Part model, mm, in its own coordinate system. A direction names the side the tool comes from. Round coordinates to 2 decimals unless told otherwise and drop trailing zeros. Write each loop counter-clockwise with the first axis right and the second up, starting at its lowest first coordinate (ties: lowest second). Pieces come first, ordered by that corner, then holes. Notation, with made-up numbers: (-38.5, 87) -> (7.5, 87) arc R9 cw to (7.5, 92) -> close; hole circle Ø7 at (39.25, -15). An arc over 180 degrees is marked (long way). Return JSON: item names as keys, results as strings. Group by question number.
```python
from build123d import *

# Parameters (mm, degrees)
SKETCH3_W           = 83
SKETCH3_H           = 60
BOSS_EXTRUDE1_DEPTH = 3
SKETCH4_R           = 1.5
CUT_EXTRUDE1_DEPTH  = 3
FILLET2_R           = 3
FILLET3_R           = 3
SKETCH8_R           = 2
BOSS_EXTRUDE2_DEPTH = 6
FILLET4_R           = 3
SKETCH9_R           = 0.3
CUT_EXTRUDE2_DEPTH  = 3


with BuildPart() as part:
    # Sketch3 → Boss-Extrude1 (new body)
    with BuildSketch(Plane(origin=(0, 0, 0), x_dir=(1, 0, 0), z_dir=(0, 1, 0))):
        Rectangle(SKETCH3_W, SKETCH3_H)
    extrude(amount=BOSS_EXTRUDE1_DEPTH)

    # Sketch4 → Cut-Extrude1 (cut)
    with BuildSketch(Plane(origin=(0, 3, 0), x_dir=(1, 0, 0), z_dir=(0, 1, 0))):
        with Locations(Location((-36.5, 25, 0), (0, 0, 270))):
            Circle(SKETCH4_R)
        with Locations(Location((36.5, 25, 0), (0, 0, 270))):
            Circle(SKETCH4_R)
        with Locations(Location((36.5, -25, 0), (0, 0, 270))):
            Circle(SKETCH4_R)
        with Locations(Location((-36.5, -25, 0), (0, 0, 270))):
            Circle(SKETCH4_R)
    extrude(amount=-CUT_EXTRUDE1_DEPTH, mode=Mode.SUBTRACT)

    # Fillet2
    fillet2_edges = [part.edges().sort_by_distance(p)[0] for p in [
        (-41.5, 1.5, 30),
    ]]
    fillet(fillet2_edges, radius=FILLET2_R)

    # Fillet3
    fillet3_edges = [part.edges().sort_by_distance(p)[0] for p in [
        (-41.5, 1.5, -30),
        (41.5, 1.5, -30),
        (41.5, 1.5, 30),
    ]]
    fillet(fillet3_edges, radius=FILLET3_R)

    # Sketch8 → Boss-Extrude2 (add)
    with BuildSketch(Plane(origin=(0, 0, 0), x_dir=(-1, 0, 0), z_dir=(0, -1, 0))):
        with Locations(Location((27.892503865, -25.595481363, 0), (0, 0, 90))):
            Circle(SKETCH8_R)
        with Locations(Location((-32.019288728, -24.830385061, 0), (0, 0, 90))):
            Circle(SKETCH8_R)
        with Locations(Location((-32.019288728, 24.653970247, 0), (0, 0, 90))):
            Circle(SKETCH8_R)
        with Locations(Location((27.892503865, 24.404518637, 0), (0, 0, 90))):
            Circle(SKETCH8_R)
    extrude(amount=BOSS_EXTRUDE2_DEPTH)

    # Fillet4
    fillet4_edges = [part.edges().sort_by_distance(p)[0] for p in [
        (-27.892503865, 0, -22.404518637),
    ]]
    fillet(fillet4_edges, radius=FILLET4_R)
    fillet4_2_edges = [part.edges().sort_by_distance(p)[0] for p in [
        (-27.892503865, 0, 27.595481363),
    ]]
    fillet(fillet4_2_edges, radius=FILLET4_R)
    # the kernel refuses this fillet: 3 mm, written as the material it adds along each edge
    with BuildSketch(Plane(origin=(32.019288728, 0, 24.830385061), x_dir=(0, 0, -1), z_dir=(-1, 0, 0))) as fillet4_3_piece_1_section:
        with BuildLine():
            CenterArc((2 + FILLET4_R, FILLET4_R), FILLET4_R, 180, 90)
            Line((2, FILLET4_R), (2 - FILLET4_R * 0.02, FILLET4_R))
            Line((2 - FILLET4_R * 0.02, FILLET4_R), (2 - FILLET4_R * 0.02, -FILLET4_R * 0.02))
            Line((2 - FILLET4_R * 0.02, -FILLET4_R * 0.02), (2 + FILLET4_R, -FILLET4_R * 0.02))
            Line((2 + FILLET4_R, -FILLET4_R * 0.02), (2 + FILLET4_R, 0))
        make_face()
    fillet4_3_piece_1 = revolve(axis=Axis((32.019288728, 0, 24.830385061), (0, -1, 0)), mode=Mode.PRIVATE)
    fillet4_3_piece_1 = fillet4_3_piece_1 - Plane(origin=(36.5, -0.855015512, 25), x_dir=(0, 0, 1), z_dir=(0, 1, 0)) * Cylinder(1.5, 21, mode=Mode.PRIVATE)
    add(fillet4_3_piece_1)
    # the kernel refuses this fillet: 3 mm, written as the material it adds along each edge
    with BuildSketch(Plane(origin=(32.019288728, 0, -24.653970247), x_dir=(0, 0, -1), z_dir=(-1, 0, 0))) as fillet4_4_piece_1_section:
        with BuildLine():
            CenterArc((2 + FILLET4_R, FILLET4_R), FILLET4_R, 180, 90)
            Line((2, FILLET4_R), (2 - FILLET4_R * 0.02, FILLET4_R))
            Line((2 - FILLET4_R * 0.02, FILLET4_R), (2 - FILLET4_R * 0.02, -FILLET4_R * 0.02))
            Line((2 - FILLET4_R * 0.02, -FILLET4_R * 0.02), (2 + FILLET4_R, -FILLET4_R * 0.02))
            Line((2 + FILLET4_R, -FILLET4_R * 0.02), (2 + FILLET4_R, 0))
        make_face()
    fillet4_4_piece_1 = revolve(axis=Axis((32.019288728, 0, -24.653970247), (0, -1, 0)), mode=Mode.PRIVATE)
    fillet4_4_piece_1 = fillet4_4_piece_1 - Plane(origin=(36.5, -0.855011953, -25), x_dir=(0, 0, 1), z_dir=(0, 1, 0)) * Cylinder(1.5, 21, mode=Mode.PRIVATE)
    add(fillet4_4_piece_1)

    # Sketch9 → Cut-Extrude2 (cut)
    with BuildSketch(Plane(origin=(0, -6, 0), x_dir=(-1, 0, 0), z_dir=(0, -1, 0))):
        with Locations(Location((27.961748008, -25.447836909, 0), (0, 0, 90))):
            Circle(SKETCH9_R)
        with Locations(Location((-32.019288728, 24.653970247, 0), (0, 0, 90))):
            Circle(SKETCH9_R)
        with Locations(Location((27.892503865, 24.404518637, 0), (0, 0, 90))):
            Circle(SKETCH9_R)
        with Locations(Location((-32.019288728, -24.830385061, 0), (0, 0, 90))):
            Circle(SKETCH9_R)
    extrude(amount=-CUT_EXTRUDE2_DEPTH, mode=Mode.SUBTRACT)


solid = part.part
```
Item 1: Two-plate mould, pull along X, no slides. Class faces 1 (the face through (-41.5, 1, 0)), 2 (the face through (40.6, 1.52, -29.14)), 3 (the face through (-29.845, -4.438, 26.029)): released by +X, released by -X, zero draft, split by the parting line, or undercut.
Item 2: Wall check: L1, parallel to X at y = 0.75, z = -25; L2, parallel to Y at x = -7, z = 10; L3, parallel to X at y = -3, z = 26. Give the ranges that are in metal, low to high.
Item 3: Cut at A-A (x = -36.5). Write the cut outline in (y, z).
Item 4: Cut at B-B (y = -4.5). Write the cut outline in (x, z), then the cut area to 3 significant figures.
Item 5: Cut at D-D (x = -17). Write the cut outline in (y, z), then the cut area to 3 significant figures.
Item 6: Which spindle directions (+Z, -Z, +X, -X, +Y, -Y) get a long thin tool onto all of the face, cutting with end or side? Do faces 4 (the face through (32, -6, 24)), 5 (the face through (30.067, -4.479, -24.22)). Say none if no direction does.
Item 7: Cut at C-C (z = 1). Write the cut outline in (x, y).
Item 8: Flat gauge pins, fed straight in: P1, Ø1, axis at x = 21, y = -1, coming from the +Z side; P2, Ø0.7, axis at x = 32, z = 25, coming from the -Y side; P3, Ø5, axis at x = -36.5, z = 25, coming from the -Y side. Where does each tip first touch, or does it go through?
Checks:
{
 "1": {"face 1": "released by -X", "face 2": "released by +X", "face 3": "undercut"},
 "2": {"L1": "x = -41.5 to -38, -35 to 35, 38 to 41.5", "L2": "y = 0 to 3", "L3": "x = -29.85 to -25.93, 30.4 to 33.64"},
 "3": {"outline": "(0, -30) -> (3, -30) -> (3, -26.5) -> (0, -26.5) -> close; (0, -23.5) -> (3, -23.5) -> (3, 23.5) -> (0, 23.5) -> close; (0, 26.5) -> (3, 26.5) -> (3, 30) -> (0, 30) -> close"},
 "4": {"outline": "circle Ø4 at (-27.89, -24.4); circle Ø4 at (-27.89, 25.6); circle Ø4 at (32.02, -24.65); circle Ø4 at (32.02, 24.83); hole circle Ø0.6 at (-27.96, 25.45); hole circle Ø0.6 at (-27.89, -24.4); hole circle Ø0.6 at (32.02, -24.65); hole circle Ø0.6 at (32.02, 24.83)", "area": "49.1 mm2"},
 "5": {"outline": "(0, -30) -> (3, -30) -> (3, 30) -> (0, 30) -> close", "area": "180 mm2"},
 "6": {"face 4": "+Z, -Z, +X, -X, -Y", "face 5": "-Y"},
 "7": {"outline": "(-41.5, 0) -> (41.5, 0) -> (41.5, 3) -> (-41.5, 3) -> close"},
 "8": {"P1": "passes through", "P2": "stops at y = -6", "P3": "stops at y = 0"}
}
